The model under review builds one solid part; all positions refer to its coordinate system, in mm. A direction names the side the tool comes from. Coordinates: 2 decimals unless noted, no trailing zeros. Order: outer loops, then holes, each group sorted by start corner. A loop starts at its lowest first (then second) coordinate and runs counter-clockwise, first axis right, second up. Notation, with made-up numbers: M 52.5,84.25 L 76.5,84.25 A14 ccw 76.5,98.25 Z; hole C 73.25,50.25 d6. An arc over 180 degrees is marked long. Write each question's results on one line, items separated by ' | '.
from build123d import *

# Parameters (mm, degrees)
EXTRUDE_1_DEPTH     = 2
SKETCH_2_R          = 1.55
CUT_EXTRUDE_1_DEPTH = 5
SKETCH_3_R          = 3
CUT_EXTRUDE_2_DEPTH = 10


with BuildPart() as part:
    # 草图1 → 凸台-拉伸1 (new body)
    with BuildSketch(Plane.XY):
        Polygon((16.974358974, 15.205128205), (16.974358974, 42.205128205), (2.974358974, 42.205128205), (-5.298152288, 42.205128205), (-10.025641026, 42.205128205), (-10.025641026, 40.205128205), (-20.025641026, 40.205128205), (-20.025641026, 42.205128205), (-47.025641026, 42.205128205), (-47.025641026, 15.205128205), (-45.025641026, 15.205128205), (-45.025641026, 5.205128205), (-47.025641026, 5.205128205), (-47.025641026, -21.794871795), (-20.025641026, -21.794871795), (-20.025641026, -19.794871795), (-10.025641026, -19.794871795), (-10.025641026, -21.794871795), (16.974358974, -21.794871795), (16.974358974, 5.205128205), align=None)
    extrude(amount=EXTRUDE_1_DEPTH)

    # 草图2 → 切除-拉伸1 (cut)
    with BuildSketch(Plane.XY):
        with Locations((-15.025641026, 10.205128205)):
            Circle(SKETCH_2_R)
    extrude(amount=CUT_EXTRUDE_1_DEPTH, mode=Mode.SUBTRACT)

    # 草图3 → 切除-拉伸2 (cut)
    with BuildSketch(Plane.XY.offset(2)):
        with Locations((0, 10.205128205)):
            Circle(SKETCH_3_R)
    extrude(amount=-CUT_EXTRUDE_2_DEPTH, mode=Mode.SUBTRACT)


solid = part.part
1) Take a section at B-B on z = 1.4. State the section outline as (x, y) points.
Solutions:
outline: M -47.03,-21.79 L -20.03,-21.79 L -20.03,-19.79 L -10.03,-19.79 L -10.03,-21.79 L 16.97,-21.79 L 16.97,42.21 L -10.03,42.21 L -10.03,40.21 L -20.03,40.21 L -20.03,42.21 L -47.03,42.21 L -47.03,15.21 L -45.03,15.21 L -45.03,5.21 L -47.03,5.21 Z; hole C -15.03,10.21 d3.1; hole C 0,10.21 d6
2) The part is to be moulded in two halves that separate along Y. For faces 4 (the flat face through (-33, 42.205, 1)), 5 (the flat face through (-23, 11, 2)), 6 (the flat face through (-46, 15.205, 1)), 7 (the cylindrical face through (-2.211, 12.233, 1.014)), say which applies: pulls with the +Y half, pulls with the -Y half, needs draft (parallel to the pull), parting line crosses it, or undercut.
Solutions:
face 4: pulls with the +Y half | face 5: needs draft | face 6: undercut | face 7: undercut
3) For pin 1 (1 mm diameter, centred on x = -13.5, z = 1, fed in from +Y); pin 2 (0.6 mm diameter, centred on y = 9.5, z = 1, fed in from -X), all flat-tipped, find the tip position at first contact; note any pin that passes through.
Solutions:
pin 1: y = 40.21 | pin 2: x = -45.03
4) To check wall thickness, follow line 1 along Y through (x, z) = (0, 0.75); line 2 along Y through (x, z) = (-11.5, 0.8). State the ranges of each line that lie inside material, in increasing order.
Solutions:
line 1: -21.79 to 7.21, 13.21 to 42.21 | line 2: -19.79 to 40.21
5) Take a section at A-A on x = 0. State the section outline as (y, z) points, plus the area to 3 significant figures.
Solutions:
outline: M -21.79,0 L 7.21,0 L 7.21,2 L -21.79,2 Z; M 13.21,0 L 42.21,0 L 42.21,2 L 13.21,2 Z | area: 116 mm2
6) Take a section at C-C on x = -11. State the section outline as (y, z) points.
Solutions:
outline: M -19.79,0 L 40.21,0 L 40.21,2 L -19.79,2 Z
7) For faces 1 (the flat face through (-45.026, 10, 1)), 2 (the flat face through (-15, 40.205, 1)), 3 (the flat face through (-15, -19.795, 1)), list the 3-axis set-ups (+Z, -Z, +X, -X, +Y, -Y) from which the entire face can be reached by the end or side of a thin tool; tool diameter is ignored.
Solutions:
face 1: +Z, -Z, -X | face 2: +Z, -Z, +Y | face 3: +Z, -Z, -Y
